Geometry check sheet. Reference: the model listing, model coordinates, mm. A direction names the side the tool comes from. Coordinates: 2 decimals unless noted, no trailing zeros. Write each loop counter-clockwise with the first axis right and the second up, starting at its lowest first coordinate (ties: lowest second). Pieces come first, ordered by that corner, then holes.
from build123d import *

# Parameters (mm, degrees)
CROQUIS2_R                   = 2.4
SALIENTE_EXTRUIR1_DEPTH      = 18.25
CORTAR_EXTRUIR_L_MINA1_DEPTH = 14.5


with BuildPart() as part:
    # Croquis2 → Saliente-Extruir1 (new, symmetric)
    with BuildSketch(Plane(origin=(0, 0, 0), x_dir=(1, 0, 0), z_dir=(0, 1, 0))):
        with Locations(Location((0, 0, 0), (0, 0, 270))):
            Circle(CROQUIS2_R)
    extrude(amount=SALIENTE_EXTRUIR1_DEPTH, both=True)

    # Croquis3 → Cortar-Extruir-Lámina1 (cut)
    with BuildSketch(Plane(origin=(0, 18.25, 0), x_dir=(1, 0, 0), z_dir=(0, 1, 0))):
        with BuildLine():
            Line((-11.75, 3.962007067), (-11.75, -3.962007067))
            ThreePointArc((-11.75, -3.962007067), (0, -12.4), (11.75, -3.962007067))
            Line((11.75, -3.962007067), (11.75, 3.962007067))
            ThreePointArc((11.75, 3.962007067), (0, 12.4), (-11.75, 3.962007067))
        make_face()
        with BuildLine():
            Line((-1.75, 1.642406771), (-1.75, -1.642406771))
            ThreePointArc((-1.75, -1.642406771), (0, -2.4), (1.75, -1.642406771))
            Line((1.75, -1.642406771), (1.75, 1.642406771))
            ThreePointArc((1.75, 1.642406771), (0, 2.4), (-1.75, 1.642406771))
        make_face(mode=Mode.SUBTRACT)
    extrude(amount=-CORTAR_EXTRUIR_L_MINA1_DEPTH, mode=Mode.SUBTRACT)


solid = part.part
1. Gauge pin test, flat end, axial feed: pin 1 Ø2 at (y, z) = (12, 1.5) entering from -X. Record the tip position at first contact, or that the pin passes through.
Computed values:
pin 1: stops at x = -1.75
2. Access from +Z, -Z, +X, -X, +Y, -Y to the whole of each face (thin tool, end or side, straight path). Record for faces 1 (the flat face through (-1.75, 11, 0)), 2 (the flat face through (1.75, 11, 0)), 3 (the flat face through (0, 18.25, 0)).
Computed values:
face 1: +Z, -Z, -X, +Y
face 2: +Z, -Z, +X, +Y
face 3: +Z, -Z, +X, -X, +Y
3. Sectioned sample at C-C, the plane x = -0.8. Record the boundary of the cut face in (y, z), and give its area (3 significant figures).
Computed values:
outline: (-18.25, -2.26) - (18.25, -2.26) - (18.25, 2.26) - (-18.25, 2.26) - close
area: 165 mm2
4. Sectioned sample at B-B, the plane y = -4.5. Record the boundary of the cut face in (x, z).
Computed values:
outline: circle Ø4.8 at (0, 0)
5. Sectioned sample at D-D, the plane y = 9.5. Record the boundary of the cut face in (x, z).
Computed values:
outline: (-1.75, -1.64) arc R2.4 ccw to (1.75, -1.64) - (1.75, 1.64) arc R2.4 ccw to (-1.75, 1.64) - close
6. Sectioned sample at A-A, the plane z = 0. Record the boundary of the cut face in (x, y).
Computed values:
outline: (-2.4, -18.25) - (2.4, -18.25) - (2.4, 3.75) - (1.75, 3.75) - (1.75, 18.25) - (-1.75, 18.25) - (-1.75, 3.75) - (-2.4, 3.75) - close
7. Thickness scan on line 1 along Z through (x, y) = (-0.1, 9); line 2 along X through (y, z) = (-1, -1.75); line 3 along X through (y, z) = (11, -1.25). Record the ranges inside material, lowest first.
Computed values:
line 1: z = -2.4 to 2.4
line 2: x = -1.64 to 1.64
line 3: x = -1.75 to 1.75
